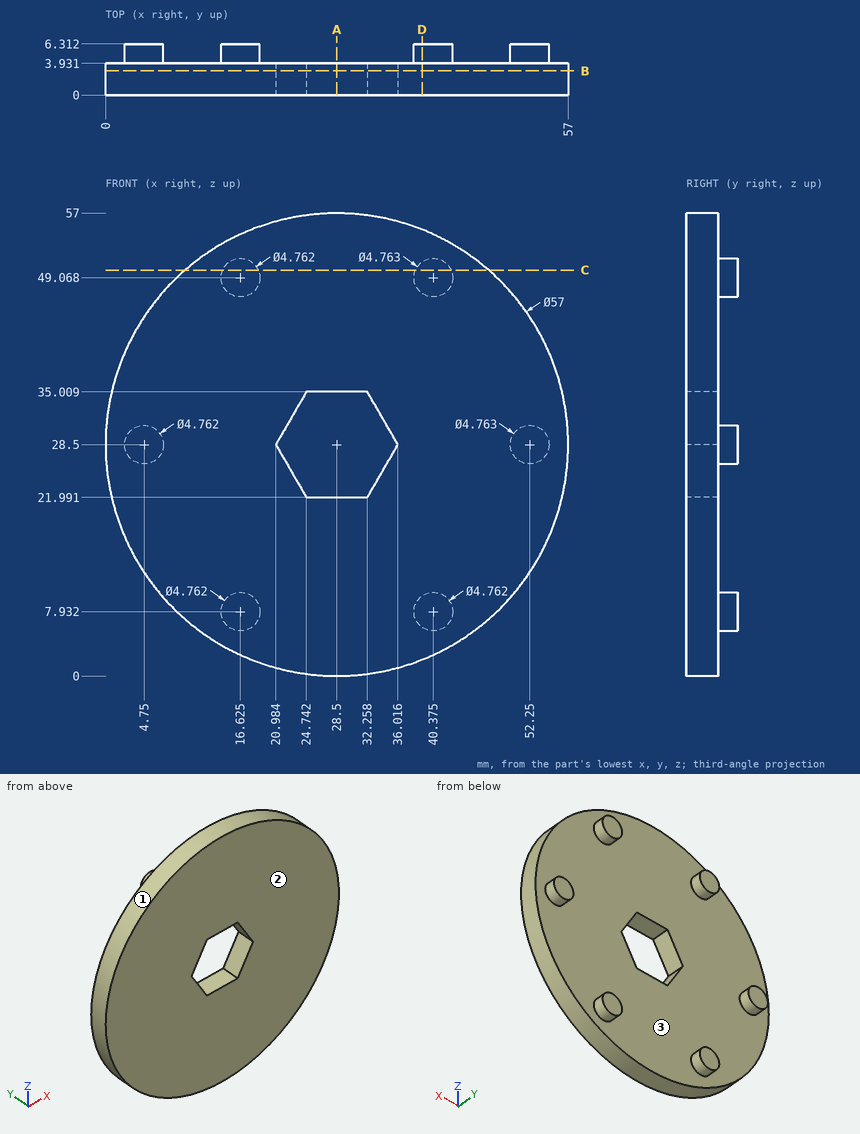
For this review, use the dimensioned drawing (mm, ordinates from the lowest corner) and the shaded views. Give positions to 0.01 mm unless a question says otherwise; leave off trailing zeros. Write each loop counter-clockwise with the first axis right and the second up, starting at its lowest first coordinate (ties: lowest second). Pieces come first, ordered by that corner, then holes. Notation, with made-up numbers: M 10.5,-13 L 21.5,-13 A34 cw 21.5,19 Z; hole C 9.25,41 d9. An arc over 180 degrees is marked long. Answer as a JSON object with one key per item and string values. Group by question number.
1) We need section A-A (x = 28.5). Give the boundary of the cut face in (y, z).
2) We need section D-D (x = 39). Give the boundary of the cut face in (y, z) (1 decimal), and give its area (3 significant figures).
3) Mouldability with a two-part tool opening along Z and no side actions: class the marked faces 1, 2 and 3 as released by +Z, released by -Z, zero draft, split by the parting line, or undercut.
4) We need section C-C (z = 50). Give the boundary of the cut face in (x, y).
5) Clearance check with flat-ended pins moving along their axes: pin 1 Ø3 at (x, y) = (28.5, 1) entering from +Z; pin 2 Ø10 at (x, z) = (31, 50) entering from +Y; pin 3 Ø2 at (x, y) = (29.5, 3) entering from -Z. State where each tip first meets the part, or that it passes through.
6) For line 1 along Y through (x, z) = (41, 19); line 2 along X through (y, z) = (4, 7) (1 decimal); line 3 along Z through (x, y) = (31.5, 2.5), list the stretches that pass through material, from the lowest coordinate up.
7) We need section B-B (y = 3). Give the boundary of the cut face in (x, z) (1 decimal).
Answer key:
{
 "1": {"outline": "M 0,0 L 3.93,0 L 3.93,21.99 L 0,21.99 Z; M 0,35.01 L 3.93,35.01 L 3.93,57 L 0,57 Z"},
 "2": {"outline": "M 0,2 L 3.9,2 L 3.9,6 L 6.3,6 L 6.3,9.9 L 3.9,9.9 L 3.9,47.1 L 6.3,47.1 L 6.3,51 L 3.9,51 L 3.9,55 L 0,55 Z", "area": "227 mm²"},
 "3": {"face 1": "split by the parting line", "face 2": "zero draft", "face 3": "undercut"},
 "4": {"outline": "M 9.79,0 L 47.21,0 L 47.21,3.93 L 42.57,3.93 L 42.57,6.31 L 38.18,6.31 L 38.18,3.93 L 18.82,3.93 L 18.82,6.31 L 14.43,6.31 L 14.43,3.93 L 9.79,3.93 Z"},
 "5": {"pin 1": "stops at z = 57", "pin 2": "stops at y = 3.93", "pin 3": "stops at z = 0"},
 "6": {"line 1": "y = 0 to 3.93", "line 2": "x = 14.4 to 18.8, 38.2 to 42.6", "line 3": "z = 0.16 to 21.99, 35.01 to 56.84"},
 "7": {"outline": "C 28.5,28.5 d57; hole M 21,28.5 L 24.7,22 L 32.3,22 L 36,28.5 L 32.3,35 L 24.7,35 Z"}
}
